Geometry check sheet. Reference: the model listing, model coordinates, mm. Face numbers are marked on the shaded views. A direction names the side the tool comes from. Round coordinates to 2 decimals unless told otherwise and drop trailing zeros. Order: outer loops, then holes, each group sorted by start corner. A loop starts at its lowest first (then second) coordinate and runs counter-clockwise, first axis right, second up. Notation, with made-up numbers: (-6, 21.5) - (-1, 21.5) arc R11 ccw to (-1, 36.5) - close; hole circle Ø7 at (-37.75, 17.5). An arc over 180 degrees is marked (long way). Answer as CSV lines item,"result". Start each with the question number.
Autodesk Inventor part; units mm, degrees
ref_plane "YZ Plane" through (0, 0, 0) normal (1, 0, 0) x (0, 1, 0)
ref_plane "XZ Plane" through (0, 0, 0) normal (0, 1, 0) x (-1, 0, 0)
ref_plane "XY Plane" through (0, 0, 0) normal (0, 0, 1) x (1, 0, 0)
sketch "Эскиз1" plane through (0, 0, 0) normal (0, 0, 1) x (1, 0, 0)
  line L0 (-25, -12.5) -> (-25, -8.5)
  line L1 (-15, -12.5) -> (-25, -12.5)
  line L2 (-25, -8.5) -> (-15, -8.5)
  line L3 (-15, -8.5) -> (-15, -12.5)
  point P0 (0, 0)
extrude "Выдавливание1" add sketch "Эскиз1" against normal blind 12
sketch "Эскиз2" plane through (-25, -8.5, 0) normal (0, 1, 0) x (1, 0, 0)
  line L0 (-6.047, -15.4734) -> (10, -15.4734)
  line L1 (10, -15.4734) -> (10, 0)
  line L2 (0, 0) -> (10, 0)
  line L3 (0, 0) -> (-6.047, -15.4734)
  line L4 (0, 0) -> (10, 0)
  point P0 (25, 0)
extrude "Выдавливание2" add sketch "Эскиз2" against normal blind 4
fillet "Сопряжение1" radius 2 2 edges at (-15, -10.5, 15.4734) (-31.047, -10.5, 15.4734)
properties part number "footbtn"
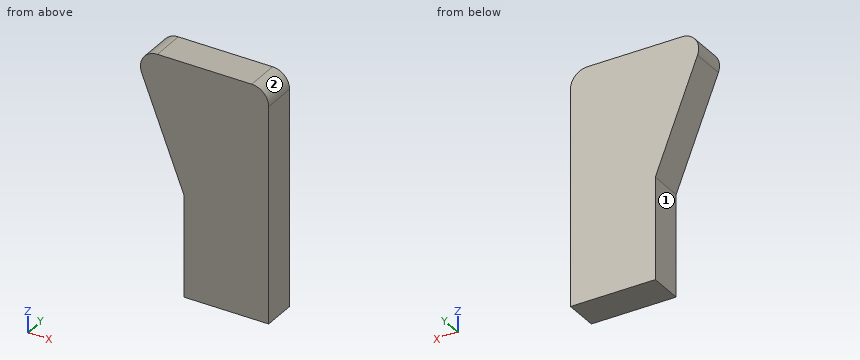
1. Section check A-A on y = -10.8. Record the boundary of the cut face in (x, z).
2. Access from +Z, -Z, +X, -X, +Y, -Y to the whole of each face (thin tool, end or side, straight path). Record for the marked faces 1 and 2.
3. Section check C-C on x = -26.75. Record the boundary of the cut face in (y, z), plus the area to 3 significant figures.
4. Thickness scan on probe 1 along X at (y, z) = (-9.2, -8.5); probe 2 along Z at (x, y) = (-16.5, -10.95); probe 3 along X at (y, z) = (-10.8, 4.5). Record the ranges inside material, lowest first.
5. Section check B-B on z = -9.5. Record the boundary of the cut face in (x, y).
Numbers:
1,outline,"(-29.98, 12.75) - (-25, 0) - (-25, -12) - (-15, -12) - (-15, 13.47) arc R2 ccw to (-17, 15.47) - (-28.12, 15.47) arc R2 ccw to start"
2,face 1,"-Z, -X, +Y, -Y"
2,face 2,"+Z, +X, +Y, -Y"
3,outline,"(-12.5, 4.48) - (-8.5, 4.48) - (-8.5, 15.47) - (-12.5, 15.47) - close"
3,area,"44.0 mm2"
4,probe 1,"x = -25 to -15"
4,probe 2,"z = -12 to 15.41"
4,probe 3,"x = -26.76 to -15"
5,outline,"(-25, -12.5) - (-15, -12.5) - (-15, -8.5) - (-25, -8.5) - close"
